from build123d import *

# Parameters (mm, degrees)
F1_DEPTH  = 2.5
F2_W      = 24
F2_H      = 6
F3_DEPTH  = 26.55
F5_DEPTH  = 33.251
F6_W      = 1.5
F6_H      = 7
F7_DEPTH  = 7
F8_R      = 2
F9_DEPTH  = 25
F11_DEPTH = 3
F12_DEPTH = 0.8


with BuildPart() as f1:
    # F0 (on Top) → F1 (new body)
    with BuildSketch(Plane.XY):
        Polygon((-7.895649, 0), (-7.895649, 27.25), (9.354351, 27.25), (9.354351, 0), (12.729351, 0), (12.729351, 33.25), (-11.270649, 33.25), (-11.270649, 0), align=None)
    extrude(amount=F1_DEPTH)

    # F2 (on face) → F3 (join)
    with BuildSketch(Plane(origin=(0, 0, 0), x_dir=(1, 0, 0), z_dir=(0, 0, -1))):
        with Locations((0.729351, -30.25)):
            Rectangle(F2_W, F2_H)
    extrude(amount=F3_DEPTH)

    # F4 (on face) → F5 (cut, through all)
    with BuildSketch(Plane(origin=(0, 33.25, 0), x_dir=(-1, 0, 0), z_dir=(0, 1, 0))):
        Polygon((11.270649, -26.55), (11.270649, 0), (-7.354351, -26.55), align=None)
    extrude(amount=-F5_DEPTH, mode=Mode.SUBTRACT)

    # F6 (on face) → F7 (join)
    with BuildSketch(Plane.XZ.offset(-27.25)):
        with Locations((8.104351, -23.05)):
            Rectangle(F6_W, F6_H)
    extrude(amount=F7_DEPTH)

    # F8 (on face) → F9 (cut)
    with BuildSketch(Plane(origin=(7.354351, 0, 0), x_dir=(0, -1, 0), z_dir=(-1, 0, 0))):
        with Locations((-23.75, -23.05)):
            Circle(F8_R)
    extrude(amount=-F9_DEPTH, mode=Mode.SUBTRACT)

    # F10 (on face) → F11 (cut)
    with BuildSketch(Plane(origin=(0, 33.25, 0), x_dir=(-1, 0, 0), z_dir=(0, 1, 0))):
        Polygon((-7.354351, -26.55), (11.270649, 0), (11.270649, 2.5), (-10.580134, 2.5), (-10.580134, -26.55), align=None)
    extrude(amount=-F11_DEPTH, mode=Mode.SUBTRACT)

    # F6 (on face) → F12 (cut)
    with BuildSketch(Plane.XZ.offset(-27.25)):
        Polygon((-11.270649, 0), (7.354351, -26.55), (7.354351, -19.55), (8.854351, -19.55), (8.854351, -26.55), (12.729351, -26.55), (12.729351, 0), (9.354351, 0), (9.354351, 2.5), (-7.895649, 2.5), (-7.895649, 0), align=None)
    extrude(amount=-F12_DEPTH, mode=Mode.SUBTRACT)

    # F13: F1 across face


with BuildPart() as f1_1:
    add(f1.part)
    add(f1.part.mirror(Plane(origin=(-9.583149, 0, 1.25), x_dir=(1, 0, 0), z_dir=(0, -1, 0))))


solid = f1_1.part
The listing builds one solid part. Answer for the finished solid, in the listing's coordinates (mm). A direction names the side the tool comes from. Give positions to 0.01 mm unless a question says otherwise; leave off trailing zeros. Write each loop counter-clockwise with the first axis right and the second up, starting at its lowest first coordinate (ties: lowest second). Pieces come first, ordered by that corner, then holes.
Item 1: Which of the six approach directions +Z, -Z, +X, -X, +Y, -Y give full straight-line access (tool end or side, diameter ignored) to faces 4 (the flat face through (8, -24, -19.55)), 5 (the flat face through (-7.896, 0, 1)), 6 (the flat face through (8, -20.25, -23))?
Item 2: Section D-D, the plane y = 26.5 is taken. Write down the section's boundary in (x, z), plus the area to 3 significant figures.
Item 3: Flat-ended cylindrical pins translate along their axes: P1, Ø1.5, axis at x = -2, z = -12.5, coming from the -Y side; P2, Ø3, axis at x = -4.5, y = -1, coming from the -Z side; P3, Ø3.5, axis at y = 31.5, z = -7.5, coming from the -X side; P4, Ø1.7, axis at x = -10, y = -1.5, coming from the -Z side. Find the tip coordinate at first contact, or state that the pin passes through.
Item 4: Section C-C, the plane z = -18.5 is taken. Write down the section's boundary in (x, y).
Item 5: Section A-A, the plane y = -7.5 is taken. Write down the section's boundary in (x, z), plus the area to 3 significant figures.
Item 6: Determine the mould class of faces 1 (the flat face through (12, -33.25, -12)), 2 (the flat face through (10.58, 32, -12)), 3 (the cylindrical face through (8.094, 25.337, -24.267)) for opening direction Y: released by +Y, released by -Y, zero draft, split by the parting line, or undercut.
Item 7: Find the intervals of material crossed by line 1 along Z through (x, y) = (8, -23.75); line 2 along Y through (x, z) = (5.75, -4); line 3 along Z through (x, y) = (11, 14), in increasing order.
Item 8: Section B-B, the plane x = 1.5 is taken. Write down the section's boundary in (y, z).
Completed:
1. face 4: +Z, +X, -X
1. face 5: +Z, -Z
1. face 6: +Z, -Z, +X, -X
2. outline: (-11.27, 0) - (-7.9, 0) - (-7.9, 2.5) - (-11.27, 2.5) - close; (7.35, -26.55) - (8.85, -26.55) - (8.85, -19.55) - (7.35, -19.55) - close; (9.35, 0) - (12.73, 0) - (12.73, 2.5) - (9.35, 2.5) - close
2. area: 27.4 mm2
3. P1: stops at y = -30.25
3. P2: passes through
3. P3: stops at x = -6.87
3. P4: stops at z = 0
4. outline: (1.71, -30.25) - (10.58, -30.25) - (10.58, -33.25) - (12.73, -33.25) - (12.73, -28.05) - (1.71, -28.05) - close; (1.71, 28.05) - (12.73, 28.05) - (12.73, 33.25) - (10.58, 33.25) - (10.58, 30.25) - (1.71, 30.25) - close
5. outline: (-11.27, 0) - (-7.9, 0) - (-7.9, 2.5) - (-11.27, 2.5) - close; (9.35, 0) - (12.73, 0) - (12.73, 2.5) - (9.35, 2.5) - close
5. area: 16.9 mm2
6. face 1: released by -Y
6. face 2: zero draft
6. face 3: undercut
7. line 1: z = -26.55 to -25.05, -21.05 to -19.55
7. line 2: y = -30.25 to -28.05, 28.05 to 30.25
7. line 3: z = 0 to 2.5
8. outline: (-30.25, -18.2) - (-28.05, -18.2) - (-28.05, 2.5) - (-30.25, 2.5) - close; (28.05, -18.2) - (30.25, -18.2) - (30.25, 2.5) - (28.05, 2.5) - close
